```python
from build123d import *

# Parameters (mm, degrees)
CUT_EXTRUDE_1_DEPTH      = 45.054236589
CUT_EXTRUDE_1_DEPTH_BACK = 45.054236589
SKETCH_2_W               = 30
SKETCH_2_H               = 10
SKETCH_3_R               = 3
CUT_EXTRUDE_2_DEPTH      = 43.296024461
SKETCH_5_R               = 10
EXTRUDE_1_DEPTH          = 9
CUT_EXTRUDE_7_DEPTH      = 43.296024461
CUT_EXTRUDE_7_DEPTH_BACK = 43.296024461
SKETCH_6_R               = 4.1
FILLET_2_R               = 5
CUT_EXTRUDE_8_DEPTH      = 4
CUT_EXTRUDE_8_DEPTH_BACK = 12


with BuildPart() as part:
    # 草图1 → 旋转2 (revolve)
    with BuildSketch(Plane.XY, mode=Mode.PRIVATE) as revolve_2_sk:
        Polygon((0, 0), (0, 8.411697794), (28.531695489, 17.682207625), (28.531695489, 9.270509831), align=None)
    revolve(revolve_2_sk.sketch.rotate(Axis((0, 0, 0), (0, 1, 0)), 270), axis=Axis((0, 0, 0), (0, 1, 0)))

    # 草图2 → 切除-拉伸1 (cut, two sides: drawn at the far end of the back side and taken through both)
    with BuildSketch(Plane.XY.offset(-CUT_EXTRUDE_1_DEPTH_BACK)):
        Rectangle(SKETCH_2_W, SKETCH_2_H)
    extrude(amount=CUT_EXTRUDE_1_DEPTH + CUT_EXTRUDE_1_DEPTH_BACK, mode=Mode.SUBTRACT)

    # 草图3 → 切除-拉伸2 (cut, through all)
    with BuildSketch(Plane.XZ.offset(-5)):
        with Locations(Location((0, 0, 0), (0, 0, 270))):
            Circle(SKETCH_3_R)
    extrude(amount=-CUT_EXTRUDE_2_DEPTH, mode=Mode.SUBTRACT)

    # 草图5 → 凸台-拉伸1 (add)
    with BuildSketch(Plane.XZ.offset(-5)):
        with Locations(Location((0, 0, 0), (0, 0, 90))):
            Circle(SKETCH_5_R)
    extrude(amount=EXTRUDE_1_DEPTH)

    # 草图6 → 切除-拉伸7 (cut, two sides: drawn at the far end of the back side and taken through both)
    with BuildSketch(Plane(origin=(0, 5, 0), x_dir=(1, 0, 0), z_dir=(0, 1, 0)).offset(-CUT_EXTRUDE_7_DEPTH_BACK)):
        with Locations(Location((0, 0, 0), (0, 0, 270))):
            Circle(SKETCH_6_R)
    extrude(amount=CUT_EXTRUDE_7_DEPTH + CUT_EXTRUDE_7_DEPTH_BACK, mode=Mode.SUBTRACT)

    # 圆角2
    fillet_2_edges = [part.edges().sort_by_distance(p)[0] for p in [
        (0, 5, -10),
    ]]
    fillet(fillet_2_edges, radius=FILLET_2_R - 0.0001)  # a hair under: the kernel refuses the full size

    # 草图9 → 切除-拉伸8 (cut, two sides: drawn at the far end of the back side and taken through both)
    with BuildSketch(Plane(origin=(0, 10, 0), x_dir=(-1, 0, 0), z_dir=(0, -1, 0)).offset(-CUT_EXTRUDE_8_DEPTH_BACK)):
        Polygon((8.48568544, -5.999428524), (9.43850023, 4.349104898), (0.95281479, 10.348533422), (-8.48568544, 5.999428524), (-9.43850023, -4.349104898), (-0.95281479, -10.348533422), align=None)
    extrude(amount=CUT_EXTRUDE_8_DEPTH + CUT_EXTRUDE_8_DEPTH_BACK, mode=Mode.SUBTRACT)


solid = part.part
```
Build history of the part. All positions in model axes, mm. A direction names the side the tool comes from. Round coordinates to 2 decimals unless told otherwise and drop trailing zeros. Write each loop counter-clockwise with the first axis right and the second up, starting at its lowest first coordinate (ties: lowest second). Pieces come first, ordered by that corner, then holes. Notation, with made-up numbers: (85.25, 72) - (133.25, 72) arc R31 ccw to (133.25, 111) - close; hole circle Ø8 at (-30, -19.75). An arc over 180 degrees is marked (long way). Answer as CSV lines item,"result".
Q1. Drop flat-ended pins along their axis: pin 1 (10 mm diameter, centred on x = 7.5, y = 6, fed in from -Z); pin 2 (1 mm diameter, centred on y = 10, z = -8.5, fed in from -X); pin 3 (2 mm diameter, centred on x = 10.5, z = -0.5, fed in from -Y); pin 4 (15 mm diameter, centred on x = -1.5, z = 4, fed in from +Y). Give the stop position or say it passes through.
Report:
pin 1,"stops at z = -28.29"
pin 2,"stops at x = -27.39"
pin 3,"stops at y = -4"
pin 4,"stops at y = 12.24"
Q2. Tool access for faces 4 (the flat face through (-8.955, 8.935, 0.898)), 5 (the cylindrical face through (4.065, 0.93, -0.534)), 6 (the flat face through (-14.5, 5, -4.6)): list every direction of +Z, -Z, +X, -X, +Y, -Y with a clear straight run to the whole face (end or side of a thin tool).
Report:
face 4,"+Y"
face 5,"+Y, -Y"
face 6,"-Y"
Q3. Cut at D-D (y = -1.75). Write the cut outline in (x, z), and give its area (3 significant figures).
Report:
outline,"circle Ø20 at (0, 0); hole circle Ø8.2 at (0, 0)"
area,"261 mm^2"
Q4. Cut at A-A (y = 10.5). Write the cut outline in (x, z).
Report:
outline,"circle Ø57.06 at (0, 0); hole (-9.44, -4.35) - (-0.95, -10.35) - (8.49, -6) - (9.44, 4.35) - (0.95, 10.35) - (-8.49, 6) - close"
Q5. Cut at B-B (x = 0). Write the cut outline in (y, z), and give its area (3 significant figures).
Report:
outline,"(-4, -10) - (0, -10) arc R5 cw to (5, -15) - (5, -15.39) - (9.27, -28.53) - (17.68, -28.53) - (11.63, -9.91) - (6, -9.91) - (6, -4.1) - (-4, -4.1) - close; (-4, 4.1) - (6, 4.1) - (6, 9.91) - (11.63, 9.91) - (17.68, 28.53) - (9.27, 28.53) - (5, 15.39) - (5, 15) arc R5 cw to (0, 10) - (-4, 10) - close"
area,"432 mm^2"
Q6. Pull direction Z, two halves, no side cores. Call faces 1 (the flat face through (-0.1, -4, 4.3)), 2 (the flat face through (-3.7, 8.935, 8.204)), 3 (the conical face through (15.524, 5.087, -2.038)): +Z half, -Z half, draft (parallel to the pull), parting line (faces both ways), or undercut.
Report:
face 1,"draft"
face 2,"undercut"
face 3,"parting line"
Q7. Drill centre lines: probe 1 along X at (y, z) = (-0.75, 0); probe 2 along X at (y, z) = (2.5, 0); probe 3 along Y at (x, z) = (-11, -24.5). Where is each one in solid material? Low to high. Write a range as [from, to].
Report:
probe 1,"x = [-10, -4.1], [4.1, 10]"
probe 2,"x = [-10.67, -4.1], [4.1, 10.67]"
probe 3,"y = [8.73, 17.14]"
